```python
from build123d import *

# Parameters (mm, degrees)
F1_DEPTH = 10
F2_W     = 69.6255117655
F2_H     = 56.8695068359
F3_DEPTH = 5
F4_W     = 5
F4_H     = 123.7891986966
F5_DEPTH = 10


with BuildPart() as f1:
    # F0 (on Front) → F1 (new body)
    with BuildSketch(Plane.XZ):
        Polygon((126.4532655478, 59.8521605134), (-130.8932900429, 59.8521605134), (-130.8932900429, 29.4098556042), (-91.0648927093, 29.4098556042), (-91.0648927093, -2.0424388349), (-51.2364953756, -2.0424388349), (-51.2364953756, -63.9370381832), (56.8277537823, -63.9370381832), (56.8277537823, -7.0675313473), (126.4532655478, -7.0675313473), align=None)
    extrude(amount=F1_DEPTH)

    # F2 (on face) → F3 (join)
    with BuildSketch(Plane(origin=(0, 0, 0), x_dir=(-1, 0, 0), z_dir=(0, 1, 0))):
        Polygon((51.2364953756, -63.9370381832), (130.8932900429, -63.9370381832), (130.8932900429, 29.4098556042), (91.0648927093, 29.4098556042), (91.0648927093, -2.0424388349), (51.2364953756, -2.0424388349), align=None)
        with Locations((-91.640509665, -35.5022847652)):
            Rectangle(F2_W, F2_H)
        Polygon((-56.8277537823, -63.9370381832), (51.2364953756, -63.9370381832), (51.2364953756, -2.0424388349), (91.0648927093, -2.0424388349), (91.0648927093, 29.4098556042), (130.8932900429, 29.4098556042), (130.8932900429, 59.8521605134), (-126.4532655478, 59.8521605134), (-126.4532655478, -7.0675313473), (-56.8277537823, -7.0675313473), align=None)
    extrude(amount=F3_DEPTH)

    # F4 (on face) → F5 (join)
    with BuildSketch(Plane.YZ.offset(126.4532655478)):
        with Locations((2.5, -2.0424388349)):
            Rectangle(F4_W, F4_H)
    extrude(amount=F5_DEPTH)


solid = f1.part
```
Input: part model. Units: mm. Frame: model coordinates. A direction names the side the tool comes from. Give positions to 0.01 mm unless a question says otherwise; leave off trailing zeros. Write each loop counter-clockwise with the first axis right and the second up, starting at its lowest first coordinate (ties: lowest second). Pieces come first, ordered by that corner, then holes. Notation, with made-up numbers: (19, -30.5) - (28, -30.5) arc R16 cw to (28, 0.5) - close; hole circle Ø7 at (-9.75, -34). An arc over 180 degrees is marked (long way). Write item = value, one per line. Start each with the question number.
1) Cut plane C-C (y = -5). Return loops of the section in (x, z), and give its area (3 significant figures).
2) Cut plane A-A (z = -38). Return loops of the section in (x, y).
3) Cut plane D-D (z = 6). Return loops of the section in (x, y).
4) Material intervals for L1, parallel to Z at x = -116, y = -7.5; L2, parallel to X at y = -9, z = -46; L3, parallel to Y at x = -117, z = -47.5, sorted ascending. Write a range as [from, to].
5) Cut plane B-B (x = -56.5). Return loops of the section in (y, z).
6) Reachability of faces 1 (the face through (91, -5, -7.068)), 2 (the face through (126.453, -5, 27)), 3 (the face through (-91.065, -5, 14)), 4 (the face through (-130.893, 1, 11)) from +Z, -Z, +X, -X, +Y, -Y: full face, straight path, thin tool, end or side. Return the list, or none.
7) Pin query (flat end, axial travel): pin 1 (3 mm diameter, centred on y = -8, z = 36.5, fed in from +X); pin 2 (8 mm diameter, centred on y = -7, z = 16.5, fed in from -X); pin 3 (5 mm diameter, centred on x = 77.5, y = -4.5, fed in from -Z). Return the tip coordinate at first contact, or that it passes through.
Answers follow:
q1.outline = (-130.89, 29.41) - (-91.06, 29.41) - (-91.06, -2.04) - (-51.24, -2.04) - (-51.24, -63.94) - (56.83, -63.94) - (56.83, -7.07) - (126.45, -7.07) - (126.45, 59.85) - (-130.89, 59.85) - close
q1.area = 21,700 mm^2
q2.outline = (-130.89, 0) - (-51.24, 0) - (-51.24, -10) - (56.83, -10) - (56.83, 0) - (136.45, 0) - (136.45, 5) - (-130.89, 5) - close
q3.outline = (-130.89, 0) - (-91.06, 0) - (-91.06, -10) - (126.45, -10) - (126.45, 0) - (136.45, 0) - (136.45, 5) - (-130.89, 5) - close
q4.L1 = [29.41, 59.85]
q4.L2 = [-51.24, 56.83]
q4.L3 = [0, 5]
q5.outline = (-10, -2.04) - (0, -2.04) - (0, -63.94) - (5, -63.94) - (5, 59.85) - (-10, 59.85) - close
q6.face_1 = -Z, +X, -Y
q6.face_2 = +Z, -Z, +X, -Y
q6.face_3 = -Z, -X, -Y
q6.face_4 = +Z, -Z, -X, +Y, -Y
q7.pin_1 = 126.45
q7.pin_2 = -91.06
q7.pin_3 = -7.07
